Autodesk Inventor part; units mm, degrees
ref_plane "to_housing_XY" through (0, 0, 0) normal (1, 0, 0) x (0, 0, -1)
ref_plane "to_housing_YZ" through (0, 0, 0) normal (0, 0, -1) x (0, 1, 0)
ref_plane "to_housing_ZX" through (0, 0, 0) normal (0, 1, 0) x (1, 0, 0)
sketch "Sketch_1" plane through (0, 0, 0) normal (0, 0, 1) x (1, 0, 0)
  line L0 (5.7, 0) -> (0.3, 0)
  arc A0 (0, 2.8) -> (0.3, 2.5) centre (0.3, 2.8) ccw
  line L1 (0.3, 2.5) -> (5.7, 2.5)
  arc A1 (5.7, 2.5) -> (6, 2.8) centre (5.7, 2.8) ccw
  line L2 (6, 2.8) -> (6, 4.25)
  line L3 (6, 4.25) -> (5.6016, 4.25)
  line L4 (5.6016, 4.25) -> (5.6016, 8.25)
  line L5 (5.6016, 8.25) -> (6, 8.25)
  line L6 (6, 8.25) -> (6, 9.2)
  arc A2 (6, 9.2) -> (5.7, 9.5) centre (5.7, 9.2) ccw
  line L7 (5.7, 9.5) -> (0.3, 9.5)
  arc A3 (0.3, 9.5) -> (0, 9.2) centre (0.3, 9.2) ccw
  line L8 (0, 9.2) -> (0, 8.25)
  line L9 (0, 8.25) -> (0.3984, 8.25)
  line L10 (0.3984, 8.25) -> (0.3984, 4.25)
  line L11 (0.3984, 4.25) -> (0, 4.25)
  line L12 (0, 4.25) -> (0, 2.8)
revolve "Revolution1" add sketch "Sketch_1" angle 360 about axis through (5.7, 0, 0) along (1, 0, 0)
ref_plane "to_housing_XY" through (0, 0, 0) normal (1, 0, 0) x (0, 0, -1)
ref_plane "to_housing_YZ" through (0, 0, 0) normal (0, 0, -1) x (0, 1, 0)
ref_plane "to_housing_ZX" through (0, 0, 0) normal (0, 1, 0) x (1, 0, 0)
ref_plane "to_housing_center_XY" through (3, 0, 0) normal (1, 0, 0) x (0, 0, -1)
ref_plane "to_housing_center_YZ" through (3, 0, 0) normal (0, 0, -1) x (0, 1, 0)
ref_plane "to_housing_center_ZX" through (3, 0, 0) normal (0, 1, 0) x (1, 0, 0)
ref_plane "作業平面7" through (3, 0, 0) normal (1, 0, 0) x (0, 0, -1)
properties part number "C-SE635ZZ"
The model under review builds one solid part; all positions refer to its coordinate system, in mm. A direction names the side the tool comes from. Round coordinates to 2 decimals unless told otherwise and drop trailing zeros. Write each loop counter-clockwise with the first axis right and the second up, starting at its lowest first coordinate (ties: lowest second). Pieces come first, ordered by that corner, then holes. Notation, with made-up numbers: (-8, -30) - (29, -30) arc R21 ccw to (29, -25) - close; hole circle Ø9 at (54, 26). An arc over 180 degrees is marked (long way). Use one line per item in the form item = value.
Q1. Consider section C-C (x = 1.1). State the section outline as (y, z) points.
Answer key:
outline = circle Ø19 at (0, 0); hole circle Ø5 at (0, 0)
Q2. Insertion check: pin 1 Ø1.5 at (x, y) = (2.5, 7.5) entering from -Z; pin 2 Ø1.5 at (x, y) = (1, 5.5) entering from -Z; pin 3 Ø3 at (x, y) = (1.5, 7) entering from -Z. Each pin has a flat end and moves straight along its axis. Give the tip position at first contact, or say it passes through.
Answer key:
pin_1 = -6.68
pin_2 = -8.23
pin_3 = -7.75
Q3. Tool access review of faces 1 (the cylindrical face through (0.2, 7.62, -3.16)), 2 (the flat face through (0, 1, -3)), 3 (the cylindrical face through (5.798, 2.285, -3.584)): name each direction out of +Z, -Z, +X, -X, +Y, -Y from which nothing blocks a thin tool from reaching the whole face with its end or side.
Answer key:
face_1 = -X
face_2 = +Z, -Z, -X, +Y, -Y
face_3 = +X
Q4. For line 1 (Z direction, x = 0.3, y = 0); line 2 (Z direction, x = 2.05, y = 0); line 3 (Y direction, x = 5.2, z = -0.5), list the stretches that pass through material, from the lowest coordinate up. Write a range as [from, to].
Answer key:
line_1 = [-9.5, -8.25], [-4.25, -2.5], [2.5, 4.25], [8.25, 9.5]
line_2 = [-9.5, -2.5], [2.5, 9.5]
line_3 = [-9.49, -2.45], [2.45, 9.49]
Q5. Draft analysis for pull direction Y (two halves, no side actions). For faces 4 (the flat face through (0, -3, 8)), 5 (the cylindrical face through (2.96, 4.38, 8.43)), 6 (the flat face through (5.602, -4, 2)), state which applies: +Y half, -Y half, draft (parallel to the pull), parting line (faces both ways), or undercut.
Answer key:
face_4 = draft
face_5 = parting line
face_6 = undercut
